Geometry check sheet. Reference: the model listing, model coordinates, mm. A direction names the side the tool comes from. Give positions to 0.01 mm unless a question says otherwise; leave off trailing zeros. Write each loop counter-clockwise with the first axis right and the second up, starting at its lowest first coordinate (ties: lowest second). Pieces come first, ordered by that corner, then holes. Notation, with made-up numbers: (-5.75, 62.25) -> (11.25, 62.25) arc R16 ccw to (11.25, 77.25) -> close; hole circle Ø8 at (5, 79). An arc over 180 degrees is marked (long way). Write item = value, one per line. Start each with the question number.
1. Cross-section at B-B, the plane x = 1.4. Record the cut outline in (y, z), plus the area to 3 significant figures.
2. Mould release check, pull along X, two halves, no side actions. Record for faces 5 (the flat face through (-2.502, 0, 1)), 6 (the flat face through (2.159, 3, 1)), 7 (the flat face through (-0.889, -3, 1)): pulls with the +X half, pulls with the -X half, needs draft (parallel to the pull), parting line crosses it, or undercut.
3. Cross-section at A-A, the plane y = -2.5. Record the cut outline in (x, z), plus the area to 3 significant figures.
4. Set-up check for faces 1 (the flat face through (-2.159, 3, 1)), 2 (the flat face through (-2.159, -3, 1)), 3 (the flat face through (1.651, -3, 1)), 4 (the flat face through (-0.381, 3, 1)): record each of +Z, -Z, +X, -X, +Y, -Y from which the full face is reachable in a straight line by a thin tool's end or side.
5. Depth check by flat-ended pin: P1, Ø0.7, axis at y = -3, z = 0.5, coming from the -X side. Enter the tip coordinate at first touch or a pass-through.
6. Thickness scan on line 1 along X through (y, z) = (-2.25, 1.05); line 2 along Y through (x, z) = (-1.45, 1.05). Record the ranges inside material, lowest first.
Autodesk Inventor part; units mm, degrees
ref_plane "YZ Plane" through (0, 0, 0) normal (1, 0, 0) x (0, 1, 0)
ref_plane "XZ Plane" through (0, 0, 0) normal (0, 1, 0) x (-1, 0, 0)
ref_plane "XY Plane" through (0, 0, 0) normal (0, 0, 1) x (1, 0, 0)
sketch "NCV8402AD-SOIC8, NCV8402AD_162" plane through (0, 0, 0) normal (0, 0, 1) x (1, 0, 0)
  line L0 (-2.159, 2.0066) -> (-2.159, 3.302)
  line L1 (-2.159, 3.302) -> (-1.651, 3.302)
  line L2 (-1.651, 3.302) -> (-1.651, 2.0066)
  line L3 (-1.651, 2.0066) -> (-0.889, 2.0066)
  line L4 (-0.889, 2.0066) -> (-0.889, 3.302)
  line L5 (-0.889, 3.302) -> (-0.381, 3.302)
  line L6 (-0.381, 3.302) -> (-0.381, 2.0066)
  line L7 (-0.381, 2.0066) -> (0.381, 2.0066)
  line L8 (0.381, 2.0066) -> (0.381, 3.302)
  line L9 (0.381, 3.302) -> (0.889, 3.302)
  line L10 (0.889, 3.302) -> (0.889, 2.0066)
  line L11 (0.889, 2.0066) -> (1.651, 2.0066)
  line L12 (1.651, 2.0066) -> (1.651, 3.302)
  line L13 (1.651, 3.302) -> (2.159, 3.302)
  line L14 (2.159, 3.302) -> (2.159, 2.0066)
  line L15 (2.159, 2.0066) -> (2.5146, 2.0066)
  line L16 (2.5146, 2.0066) -> (2.5146, -2.0016)
  line L17 (2.5146, -2.0016) -> (2.159, -2.0016)
  line L18 (2.159, -2.0016) -> (2.159, -3.302)
  line L19 (2.159, -3.302) -> (1.651, -3.302)
  line L20 (1.651, -3.302) -> (1.651, -2.0016)
  line L21 (1.651, -2.0016) -> (0.889, -2.0016)
  line L22 (0.889, -2.0016) -> (0.889, -3.302)
  line L23 (0.889, -3.302) -> (0.381, -3.302)
  line L24 (0.381, -3.302) -> (0.381, -2.0016)
  line L25 (0.381, -2.0016) -> (-0.381, -2.0016)
  line L26 (-0.381, -2.0016) -> (-0.381, -3.302)
  line L27 (-0.381, -3.302) -> (-0.889, -3.302)
  line L28 (-0.889, -3.302) -> (-0.889, -2.0016)
  line L29 (-0.889, -2.0016) -> (-1.651, -2.0016)
  line L30 (-1.651, -2.0016) -> (-1.651, -3.302)
  line L31 (-1.651, -3.302) -> (-2.159, -3.302)
  line L32 (-2.159, -3.302) -> (-2.159, -2.0016)
  line L33 (-2.159, -2.0016) -> (-2.5016, -2.0016)
  line L34 (-2.5016, -2.0016) -> (-2.5016, 2.0066)
  line L35 (-2.5016, 2.0066) -> (-2.159, 2.0066)
extrude "Extrusion1" add sketch "NCV8402AD-SOIC8, NCV8402AD_162" along normal blind 1.48
properties part number "NCV8402AD"
Answers:
q1.outline = (-2, 0) -> (2.01, 0) -> (2.01, 1.48) -> (-2, 1.48) -> close
q1.area = 5.93 mm^2
q2.face_5 = pulls with the -X half
q2.face_6 = pulls with the +X half
q2.face_7 = undercut
q3.outline = (-2.16, 0) -> (-1.65, 0) -> (-1.65, 1.48) -> (-2.16, 1.48) -> close; (-0.89, 0) -> (-0.38, 0) -> (-0.38, 1.48) -> (-0.89, 1.48) -> close; (0.38, 0) -> (0.89, 0) -> (0.89, 1.48) -> (0.38, 1.48) -> close; (1.65, 0) -> (2.16, 0) -> (2.16, 1.48) -> (1.65, 1.48) -> close
q3.area = 3.01 mm^2
q4.face_1 = +Z, -Z, -X, +Y
q4.face_2 = +Z, -Z, -X, -Y
q4.face_3 = +Z, -Z, -Y
q4.face_4 = +Z, -Z, +Y
q5.P1 = -2.16
q6.line_1 = -2.16 to -1.65, -0.89 to -0.38, 0.38 to 0.89, 1.65 to 2.16
q6.line_2 = -2 to 2.01
